Part model, mm, in its own coordinate system. A direction names the side the tool comes from. Give positions to 0.01 mm unless a question says otherwise; leave off trailing zeros. Order: outer loops, then holes, each group sorted by start corner. A loop starts at its lowest first (then second) coordinate and runs counter-clockwise, first axis right, second up. Notation, with made-up numbers: M -38,9.25 L -3,9.25 A26 cw -3,37.25 Z; hole C 81,-23.5 d9. An arc over 180 degrees is marked long. Return JSON: item names as keys, results as strings.
from build123d import *

# Parameters (mm, degrees)
F0_W           = 42
F0_H           = 42
F1_DEPTH       = 4
F3_D           = 4
F3_DEPTH       = 55
F3_TIP         = 1.2017212381
F4_D           = 23
F4_DEPTH       = 55
F4_TIP         = 6.9098971188
F5_DEPTH       = 23
F7_D           = 6
F7_DEPTH       = 55
F7_CBORE_D     = 10
F7_CBORE_DEPTH = 2
F7_TIP         = 1.8025818571
F8_SIZE        = 2
F9_DEPTH       = 2


with BuildPart() as f1:
    # F0 (on Top) → F1 (new body)
    with BuildSketch(Plane.XY):
        Rectangle(F0_W, F0_H)
    extrude(amount=F1_DEPTH)

    # F3
    with Locations(Plane.XY.offset(4)):
        with Locations((-15.5, 15.5), (-15.5, -15.5), (15.5, 15.5), (15.5, -15.5)):
            Hole(F3_D / 2, depth=F3_DEPTH)
            with Locations((0, 0, -(F3_DEPTH + F3_TIP / 2))):  # 118° drill point
                Cone(0, F3_D / 2, F3_TIP, mode=Mode.SUBTRACT)

    # F4
    with Locations(Plane.XY.offset(4)):
        with Locations((0, 0)):
            Hole(F4_D / 2, depth=F4_DEPTH)
            with Locations((0, 0, -(F4_DEPTH + F4_TIP / 2))):  # 118° drill point
                Cone(0, F4_D / 2, F4_TIP, mode=Mode.SUBTRACT)

    # F5 (add): a face of the model
    f5_faces = [f1.faces().sort_by_distance(p)[0] for p in [
        (0, -21, 2),
    ]]
    extrude(f5_faces, amount=F5_DEPTH)

    # F7
    with Locations(Plane.XY.offset(4)):
        with Locations((-10, -34), (10, -34)):
            CounterBoreHole(F7_D / 2, F7_CBORE_D / 2, F7_CBORE_DEPTH, depth=F7_DEPTH)
            with Locations((0, 0, -(F7_DEPTH + F7_TIP / 2))):  # 118° drill point
                Cone(0, F7_D / 2, F7_TIP, mode=Mode.SUBTRACT)

    # F8
    f8_edges = [f1.edges().sort_by_distance(p)[0] for p in [
        (21, 21, 2),
        (-21, 21, 2),
    ]]
    chamfer(f8_edges, length=F8_SIZE)

    # F9 (add): a face of the model
    f9_faces = [f1.faces().sort_by_distance(p)[0] for p in [
        (0, -12.426722897, 4),
    ]]
    extrude(f9_faces, amount=F9_DEPTH)


solid = f1.part
Q1. Two-plate mould, pull along Y, no slides. Class faces 3 (the flat face through (0, -44, 3)), 4 (the flat face through (-10.1, -37.3, 2)), 5 (the flat face through (20, 20, 3)), 6 (the cylindrical face through (12.21, -31.97, 0.99)): +Y half, -Y half, draft (parallel to the pull), parting line (faces both ways), or undercut.
Established:
{"face 3": "-Y half", "face 4": "undercut", "face 5": "+Y half", "face 6": "undercut"}
Q2. Band-saw the part on B-B (y = 15.5). Give the cut face in (x, z), then the cut area to 3 significant figures.
Established:
{"outline": "M -21,0 L -17.5,0 L -17.5,6 L -21,6 Z; M -13.5,0 L 13.5,0 L 13.5,6 L -13.5,6 Z; M 17.5,0 L 21,0 L 21,6 L 17.5,6 Z", "area": "204 mm²"}
Q3. Pin check, flat tips, straight feed: pin 1 (5 mm diameter, centred on x = -10, y = -34, fed in from +Z); pin 2 (9 mm diameter, centred on x = 10, y = -34, fed in from +Z). Stop position of each tip, or through.
Established:
{"pin 1": "passes through", "pin 2": "stops at z = 2"}
Q4. 3-axis set-ups, long thin cutter, end or side, ignore diameter. For faces 1 (the cylindrical face through (15.76, -13.517, 2.958)), 2 (the flat face through (9.9, -37.3, 2)): which of +Z, -Z, +X, -X, +Y, -Y reach the whole face in a straight line?
Established:
{"face 1": "+Z, -Z", "face 2": "+Z"}
Q5. Probe line 1 along Y through (x, z) = (-15.5, 4.65); line 2 along Y through (x, z) = (10, 3.5); line 3 along Y through (x, z) = (0, 1.45). List the from-to ranges inside material, lowest first.
Established:
{"line 1": "y = -44 to -17.5, -13.5 to 13.5, 17.5 to 21", "line 2": "y = -44 to -39, -29 to -5.68, 5.68 to 21", "line 3": "y = -44 to -11.5, 11.5 to 21"}
Q6. Band-saw the part on A-A (y = 0). Give the cut face in (x, z), then the cut area to 3 significant figures.
Established:
{"outline": "M -21,0 L -11.5,0 L -11.5,6 L -21,6 Z; M 11.5,0 L 21,0 L 21,6 L 11.5,6 Z", "area": "114 mm²"}
Q7. Band-saw the part on C-C (x = 0). Give the cut face in (y, z), then the cut area to 3 significant figures.
Established:
{"outline": "M -44,0 L -11.5,0 L -11.5,6 L -44,6 Z; M 11.5,0 L 21,0 L 21,6 L 11.5,6 Z", "area": "252 mm²"}
Q8. Band-saw the part on D-D (z = 5). Give the cut face in (x, y), then the cut area to 3 significant figures.
Established:
{"outline": "M -21,-44 L 21,-44 L 21,19 L 19,21 L -19,21 L -21,19 Z; hole C -15.5,-15.5 d4; hole C -15.5,15.5 d4; hole C -10,-34 d10; hole C 0,0 d23; hole C 10,-34 d10; hole C 15.5,-15.5 d4; hole C 15.5,15.5 d4", "area": "2,100 mm²"}
